The model under review builds one solid part; all positions refer to its coordinate system, in mm. Face numbers are marked on the shaded views. A direction names the side the tool comes from. Give positions to 0.01 mm unless a question says otherwise; leave off trailing zeros. Order: outer loops, then holes, each group sorted by start corner. A loop starts at its lowest first (then second) coordinate and runs counter-clockwise, first axis right, second up.
```python
from build123d import *

# Parameters (mm, degrees)
F0_W     = 51.6930520535
F0_H     = 49.859970808
F1_DEPTH = 25.4
F2_R     = 24.929985404
F3_DEPTH = 76.2
F4_R     = 24.929985404
F5_DEPTH = 25.4
F6_R     = 7.62


with BuildPart() as f1:
    # F0 (on Front) → F1 (new body)
    with BuildSketch(Plane.XZ):
        with Locations((-5.3159445524, 147.0135599375)):
            Rectangle(F0_W, F0_H)
    extrude(amount=F1_DEPTH)

    # F2 (on face) → F3 (join)
    with BuildSketch(Plane.XZ.offset(25.4)):
        with Locations((-5.3159445524, 147.0135599375)):
            Circle(F2_R)
    extrude(amount=F3_DEPTH)

    # F4 (on face) → F5 (join)
    with BuildSketch(Plane.XZ.offset(101.6)):
        with Locations((-5.3159445524, 147.0135599375)):
            Circle(F4_R)
    extrude(amount=F5_DEPTH)

    # F6
    f6_edges = [f1.edges().sort_by_distance(p)[0] for p in [
        (-30.24593, -127, 147.01356),
    ]]
    fillet(f6_edges, radius=F6_R)


solid = f1.part
```
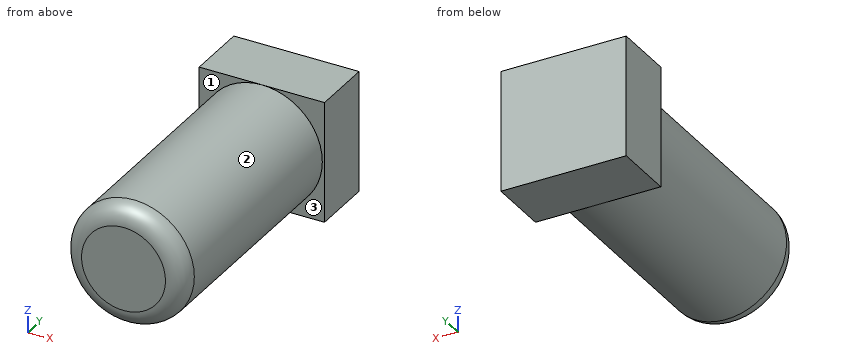
Item 1: For line 1 (X direction, y = -89.5, z = 148); line 2 (Z direction, x = -5, y = -37.5); line 3 (Y direction, x = 6.5, z = 124.5), list the stretches that pass through material, from the lowest coordinate up.
Values found:
line 1: x = -30.23 to 19.59
line 2: z = 122.09 to 171.94
line 3: y = -25.4 to 0
Item 2: Take a section at A-A (y = -93). Give the boundary of the cut face in (x, z), and give its area (3 significant figures).
Values found:
outline: circle Ø49.86 at (-5.32, 147.01)
area: 1,950 mm2
Item 3: Clearance check with flat-ended pins moving along their axes: pin 1 Ø10 at (y, z) = (-103.5, 155) entering from -X; pin 2 Ø4 at (x, z) = (4, 166) entering from -Y; pin 3 Ø3 at (y, z) = (-90, 166) entering from +X. State where each tip first meets the part, or that it passes through.
Values found:
pin 1: stops at x = -30.07
pin 2: stops at y = -126.77
pin 3: stops at x = 12.45
Item 4: For the marked faces 1, 2 and 3, list the 3-axis set-ups (+Z, -Z, +X, -X, +Y, -Y) from which the entire face can be reached by the end or side of a thin tool; tool diameter is ignored.
Values found:
face 1: -X, -Y
face 2: -Y
face 3: +X, -Y
